from build123d import *

# Parameters (mm, degrees)
SKETCH1_R           = 1.25
BOSS_EXTRUDE2_DEPTH = 20
SKETCH1_5_W         = 33
SKETCH1_5_H         = 12
SKETCH1_5_R         = 1.25
BOSS_EXTRUDE3_DEPTH = 10


with BuildPart() as part:
    # Sketch1 → Boss-Extrude2 (new body)
    with BuildSketch(Plane.XY):
        with Locations((29.04, 6)):
            Circle(SKETCH1_R)
    extrude(amount=BOSS_EXTRUDE2_DEPTH)

    # Sketch1<5> → Boss-Extrude3 (add)
    with BuildSketch(Plane.XY):
        with Locations((16.5, 6)):
            Rectangle(SKETCH1_5_W, SKETCH1_5_H)
        with Locations((29.04, 6)):
            Circle(SKETCH1_5_R, mode=Mode.SUBTRACT)
    extrude(amount=BOSS_EXTRUDE3_DEPTH)


solid = part.part
Read the model definition and answer for the solid it produces. Units are mm, in the model's axes. Give positions to 0.01 mm unless a question says otherwise; leave off trailing zeros. Write each loop counter-clockwise with the first axis right and the second up, starting at its lowest first coordinate (ties: lowest second). Pieces come first, ordered by that corner, then holes. Notation, with made-up numbers: M -11,19 L 21,19 A10 cw 21,26 Z; hole C -27,44.25 d10. An arc over 180 degrees is marked long. One line per item, written item: value. Start each with the question number.
(1) Find section D-D (y = 9.5). Determine the outline of the cut face in (x, z).
(2) Determine the mould class of faces 1 (the flat face through (16, 12, 5)), 2 (the cylindrical face through (28.05, 5.24, 14.93)), 3 (the flat face through (29, 6, 20)) for opening direction Y: pulls with the +Y half, pulls with the -Y half, needs draft (parallel to the pull), parting line crosses it, or undercut.
(3) Find section A-A (x = 29.04). Determine the outline of the cut face in (y, z).
(4) A flat-ended cylindrical pin translates along its axis: pin 1 Ø6 at (x, y) = (17.5, 2) entering from +Z. Find the tip coordinate at first contact, or state that the pin passes through.
(5) Find section C-C (z = 10.5). Determine the outline of the cut face in (x, y).
(6) Find the intervals of material crossed by line 1 (Z direction, x = 27, y = 2.75); line 2 (Y direction, x = 28.5, z = 15), in increasing order.
(7) Find section B-B (y = 6). Determine the outline of the cut face in (x, z).
Results below:
1. outline: M 0,0 L 33,0 L 33,10 L 0,10 Z
2. face 1: pulls with the +Y half
2. face 2: parting line crosses it
2. face 3: needs draft
3. outline: M 0,0 L 12,0 L 12,10 L 7.25,10 L 7.25,20 L 4.75,20 L 4.75,10 L 0,10 Z
4. pin 1: stops at z = 10
5. outline: C 29.04,6 d2.5
6. line 1: z = 0 to 10
6. line 2: y = 4.87 to 7.13
7. outline: M 0,0 L 33,0 L 33,10 L 30.29,10 L 30.29,20 L 27.79,20 L 27.79,10 L 0,10 Z
